```python
from build123d import *

# Parameters (mm, degrees)
PAD001_DEPTH           = 20
SKETCH003_R            = 2
POCKET001_DEPTH        = 4.001
LINEARPATTERN001_COUNT = 5
LINEARPATTERN001_PITCH = 11.25
POCKET002_DEPTH        = 18
FILLET_R               = 1
FILLET001_R            = 1


with BuildPart() as part:
    # Sketch002 → Pad001 (new body)
    with BuildSketch(Plane.XY):
        with BuildLine():
            Line((0, -8.676507), (-60, -8.676507))
            Line((-60, -8.676507), (-60, -10.676507))
            Line((-60, -10.676507), (0, -10.676507))
            ThreePointArc((0, -10.676507), (5.828427, -9.676507), (0, -8.676507))
        make_face()
    extrude(amount=PAD001_DEPTH)

    # Sketch003 → Pocket001 (cut, through all)
    with BuildSketch(Plane.XZ.offset(10.676507)):
        with Locations((-53, 10)):
            Circle(SKETCH003_R)
    pocket001 = extrude(amount=-POCKET001_DEPTH, mode=Mode.SUBTRACT)

    # LinearPattern001: Pocket001 ×5
    with Locations(*[(i * LINEARPATTERN001_PITCH, 0, 0) for i in range(1, LINEARPATTERN001_COUNT)]):
        add(pocket001, mode=Mode.SUBTRACT)

    # Sketch005 → Pocket002 (cut)
    with BuildSketch(Plane.XY.offset(20)):
        with BuildLine():
            ThreePointArc((5.527045, -12.375125), (6.644849, -9.676507), (5.527045, -6.97789))
            Line((4.242641, -8.262294), (5.527045, -6.97789))
            ThreePointArc((4.242641, -8.262294), (0.828427, -9.676507), (4.242641, -11.090721))
            Line((4.242641, -11.090721), (5.527045, -12.375125))
        make_face()
    extrude(amount=-POCKET002_DEPTH, mode=Mode.SUBTRACT)

    # Fillet
    fillet_edges = [part.edges().sort_by_distance(p)[0] for p in [
        (-55, -10.676507, 10),
    ]]
    fillet(fillet_edges, radius=FILLET_R)

    # Fillet001
    fillet001_edges = [part.edges().sort_by_distance(p)[0] for p in [
        (-32.5, -8.676507, 10),
    ]]
    fillet(fillet001_edges, radius=FILLET001_R)


solid = part.part
```
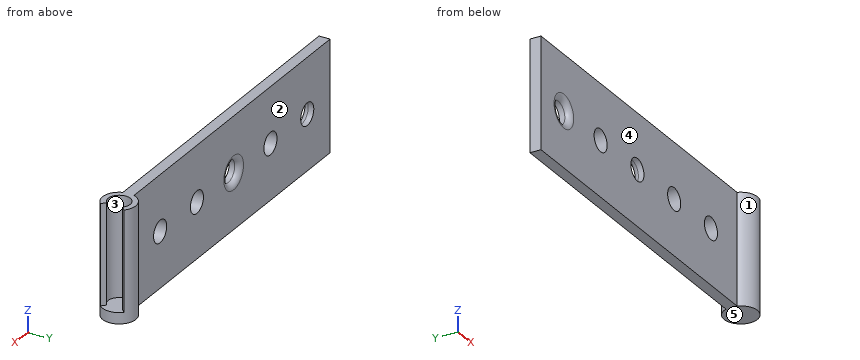
Here's how the part is built. I have some questions about the finished solid (model axes, mm). Face numbers are marked on the shaded views. A direction names the side the tool comes from. Coordinates: 2 decimals unless noted, no trailing zeros. Order: outer loops, then holes, each group sorted by start corner. A loop starts at its lowest first (then second) coordinate and runs counter-clockwise, first axis right, second up.
1) Imagine slicing it at D-D on x = -30.5. List the corners of the cut face in (y, z) for me.
2) Will these pins go through, and if not, where does the flat tip stop? pin 1 (6.5 mm diameter, centred on x = -41.75, z = 10, fed in from -Y); pin 2 (2.5 mm diameter, centred on x = -8, z = 10, fed in from +Y); pin 3 (1 mm diameter, centred on x = -17.5, z = 17, fed in from +Y).
3) Imagine slicing it at C-C on z = 3.25. List the corners of the cut face in (x, y) for me.
4) Imagine slicing it at A-A on x = -19.25. List the corners of the cut face in (y, z) for me.
5) We'd pull the mould along Y, two halves only. Please class the marked faces 1, 2 and 3: +Y half, -Y half, draft (parallel to the pull), parting line (faces both ways), or undercut.
6) Imagine slicing it at B-B on z = 10. State how many separate pieces and enclosed holes the cut face has, and give its area (3 significant figures).
7) I need wall thicknesses on line 1 (Z direction, x = -8, y = -9.85); line 2 (Y direction, x = -33, z = 17.5); line 3 (X direction, y = -11.35, z = 7.25). Which ranges of each line are inside material? Lowest first, please.
8) Which directions (+Z, -Z, +X, -X, +Y, -Y) give clear straight access to the entire face, cutting with the end or side of a thin tool? Please do the marked faces 4 and 5.
Response values:
1. outline: (-10.68, 0) - (-8.68, 0) - (-8.68, 7) arc R1 ccw to (-9.68, 8) - (-10.68, 8) - close; (-10.68, 12) - (-9.68, 12) arc R1 ccw to (-8.68, 13) - (-8.68, 20) - (-10.68, 20) - close
2. pin 1: stops at y = -10.68
2. pin 2: passes through
2. pin 3: stops at y = -8.68
3. outline: (-60, -10.68) - (0, -10.68) arc R3 ccw to (4.95, -11.8) - (4.24, -11.09) arc R2 cw (long way) to (4.24, -8.26) - (4.95, -7.56) arc R3 ccw to (0, -8.68) - (-60, -8.68) - close
4. outline: (-10.68, 0) - (-8.68, 0) - (-8.68, 8) - (-10.68, 8) - close; (-10.68, 12) - (-8.68, 12) - (-8.68, 20) - (-10.68, 20) - close
5. face 1: parting line
5. face 2: +Y half
5. face 3: undercut
6. separate pieces: 6
6. enclosed holes: 0
6. area: 90.7 mm2
7. line 1: z = 0 to 8, 12 to 20
7. line 2: y = -10.68 to -8.68
7. line 3: x = 0.34 to 1.73, 3.92 to 4.5
8. face 4: +Z, -Z, -X, -Y
8. face 5: -Z, +X, -X, +Y, -Y
